from build123d import *

# Parameters (mm, degrees)
BOSS_EXTRUDE1_DEPTH = 20
FILLET1_R           = 3
SKETCH2_R           = 2.5
CUT_EXTRUDE1_DEPTH  = 117.967247128
SKETCH3_R           = 2.5
CUT_EXTRUDE2_DEPTH  = 89.566359302
SKETCH3_4_R         = 2.5
CUT_EXTRUDE3_DEPTH  = 3.175
FILLET2_R           = 1


with BuildPart() as part:
    # Sketch1 → Boss-Extrude1 (new body)
    with BuildSketch(Plane.XY):
        with BuildLine():
            Line((5, -29.78321675), (5, -48.83321675))
            Line((5, -48.83321675), (10, -48.83321675))
            Line((10, -48.83321675), (10, -33.749666665))
            ThreePointArc((10, -33.749666665), (35.2, 0), (10, 33.749666665))
            Line((10, 33.749666665), (10, 55))
            Line((10, 55), (50, 55))
            Line((50, 55), (50, 62))
            Line((50, 62), (-50, 62))
            Line((-50, 62), (-50, 55))
            Line((-50, 55), (-10, 55))
            Line((-10, 55), (-10, 33.749666665))
            ThreePointArc((-10, 33.749666665), (-35.2, 0), (-10, -33.749666665))
            Line((-10, -33.749666665), (-10, -48.83321675))
            Line((-10, -48.83321675), (-5, -48.83321675))
            Line((-5, -48.83321675), (-5, -29.78321675))
            ThreePointArc((-5, -29.78321675), (0, 30.2), (5, -29.78321675))
        make_face()
    extrude(amount=BOSS_EXTRUDE1_DEPTH)

    # Fillet1
    fillet1_edges = [part.edges().sort_by_distance(p)[0] for p in [
        (-10, 55, 10),
        (10, 55, 10),
        (10, 33.749666665, 10),
        (-10, 33.749666665, 10),
    ]]
    fillet(fillet1_edges, radius=FILLET1_R)

    # Sketch2 → Cut-Extrude1 (cut, through all)
    with BuildSketch(Plane(origin=(0, 55, 0), x_dir=(-1, 0, 0), z_dir=(0, -1, 0))):
        with Locations(Location((40, -10, 0), (0, 0, 90))):
            Circle(SKETCH2_R)
        with Locations(Location((-40, -10, 0), (0, 0, 90))):
            Circle(SKETCH2_R)
    extrude(amount=-CUT_EXTRUDE1_DEPTH, mode=Mode.SUBTRACT)

    # Sketch3 → Cut-Extrude2 (cut, through all)
    with BuildSketch(Plane.ZY.offset(10)):
        with Locations((10, -41.83321675)):
            Circle(SKETCH3_R)
    extrude(amount=-CUT_EXTRUDE2_DEPTH, mode=Mode.SUBTRACT)

    # Sketch3_4 → Cut-Extrude3 (cut)
    with BuildSketch(Plane.ZY.offset(10)):
        Polygon((15.600297611, -41.83321675), (12.800148806, -36.98321675), (7.199851194, -36.98321675), (4.399702389, -41.83321675), (7.199851194, -46.68321675), (12.800148806, -46.68321675), align=None)
        with Locations((10, -41.83321675)):
            Circle(SKETCH3_4_R, mode=Mode.SUBTRACT)
    extrude(amount=-CUT_EXTRUDE3_DEPTH, mode=Mode.SUBTRACT)

    # Fillet2
    fillet2_edges = [part.edges().sort_by_distance(p)[0] for p in [
        (-10, -41.291441708, 20),
        (-7.5, -48.83321675, 20),
        (-5, -39.30821675, 20),
        (0, 30.2, 20),
        (5, -39.30821675, 20),
        (7.5, -48.83321675, 20),
        (10, -41.291441708, 20),
        (35.184584451, -1.041641486, 20),
        (10, 43.959955457, 20),
        (31.5, 55, 20),
        (-35.184584451, -1.041641486, 20),
        (50, 58.5, 20),
        (-10, 43.959955457, 20),
        (10.544106352, 34.196952298, 20),
        (0, 62, 20),
        (10.878679656, 54.121320344, 20),
        (-10.544106352, 34.196952298, 20),
        (-10.878679656, 54.121320344, 20),
        (-50, 58.5, 20),
        (-31.5, 55, 20),
    ]]
    fillet(fillet2_edges, radius=FILLET2_R)


solid = part.part
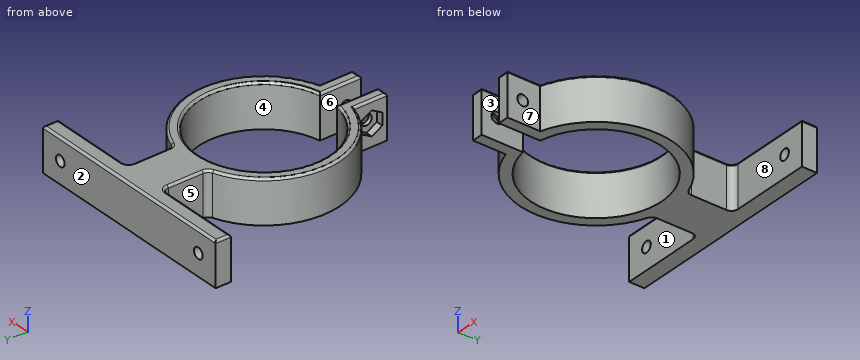
Geometry: final body of the model. Coordinates: model frame, mm. Face numbers are marked on the shaded views. A direction names the side the tool comes from. Give positions to 0.01 mm unless a question says otherwise; leave off trailing zeros. Order: outer loops, then holes, each group sorted by start corner. A loop starts at its lowest first (then second) coordinate and runs counter-clockwise, first axis right, second up. Notation, with made-up numbers: (64.25, -4.75) -> (90.25, -4.75) arc R20 ccw to (90.25, 5.25) -> close; hole circle Ø8 at (-39, 14). An arc over 180 degrees is marked (long way). Write each question's results on one line, items separated by ' | '.
1) Cut plane B-B (z = 17.75). Output: boundary loops of the cut face in (x, y).
Geometry says:
outline: (-50, 55) -> (-13, 55) arc R3 cw to (-10, 52) -> (-10, 35.92) arc R3 cw to (-11.98, 33.1) arc R35.2 ccw to (-10, -33.75) -> (-10, -48.83) -> (-5, -48.83) -> (-5, -29.78) arc R30.2 cw (long way) to (5, -29.78) -> (5, -48.83) -> (10, -48.83) -> (10, -33.75) arc R35.2 ccw to (11.98, 33.1) arc R3 cw to (10, 35.92) -> (10, 52) arc R3 cw to (13, 55) -> (50, 55) -> (50, 62) -> (-50, 62) -> close
2) Set-up query: the marked faces 5, 6, 7 and 8. Return all of +Z, -Z, +X, -X, +Y, -Y with unobstructed straight access to the full face (end or side cutting, diameter ignored); none if empty.
Geometry says:
face 5: +Z, -Z, -X | face 6: +Z, -Z, -Y | face 7: +Z, -Z, +X, -Y | face 8: +Z, -Z, +X
3) First-contact query: pin 1 Ø5.5 at (y, z) = (-41, 7.5) entering from +X; pin 2 Ø1.5 at (y, z) = (-5.5, 17) entering from +X; pin 3 Ø3 at (y, z) = (-41, 7.5) entering from -X (3 decimals). Flat tips, straight axial feed; report the tip coordinate or a pass-through.
Geometry says:
pin 1: stops at x = 10 | pin 2: stops at x = 34.88 | pin 3: stops at x = -6.825
4) Draft query along Y for the marked faces 1, 2, 3 and 4. Return one class per face: released by +Y, released by -Y, zero draft, split by the parting line, or undercut.
Geometry says:
face 1: undercut | face 2: released by +Y | face 3: zero draft | face 4: undercut
5) Cut plane A-A (x = -40). Output: boundary loops of the cut face in (y, z), and give its area (3 significant figures).
Geometry says:
outline: (55, 0) -> (62, 0) -> (62, 7.5) -> (55, 7.5) -> close; (55, 12.5) -> (62, 12.5) -> (62, 19) arc R1 ccw to (61, 20) -> (56, 20) arc R1 ccw to (55, 19) -> close | area: 105 mm²
6) Cut plane C-C (z = 10). Give the number of separate pieces and of enclosed holes in the cut face, and give its area (3 significant figures).
Geometry says:
separate pieces: 5 | enclosed holes: 0 | area: 2,100 mm²
7) Cut plane D-D (x = 0). Output: boundary loops of the cut face in (y, z).
Geometry says:
outline: (30.2, 0) -> (62, 0) -> (62, 19) arc R1 ccw to (61, 20) -> (31.2, 20) arc R1 ccw to (30.2, 19) -> close
8) Line query: line 1 along X through (y, z) = (56.5, 10); line 2 along X through (y, z) = (-1, 4.75); line 3 along Y through (x, z) = (-9.5, 6.25). Output: solid intervals per line, ascending.
Geometry says:
line 1: x = -50 to -42.5, -37.5 to 37.5, 42.5 to 50 | line 2: x = -35.19 to -30.18, 30.18 to 35.19 | line 3: y = -48.83 to -45.04, -38.63 to -28.67, 28.67 to 62
